Part model, mm, in its own coordinate system. Round coordinates to 2 decimals unless told otherwise and drop trailing zeros. Order: outer loops, then holes, each group sorted by start corner. A loop starts at its lowest first (then second) coordinate and runs counter-clockwise, first axis right, second up. Notation, with made-up numbers: (-31, 81.5) - (18, 81.5) arc R22 cw to (18, 109.5) - close; hole circle Ø5 at (79, 58). An arc over 180 degrees is marked (long way). Answer as a JSON object with one key per item and string values.
```python
from build123d import *

# Parameters (mm, degrees)
BOSS_EXTRUDE1_DEPTH = 4
SKETCH3_R           = 4
CUT_EXTRUDE1_DEPTH  = 105.985426706
FILLET1_R           = 5


with BuildPart() as part:
    # Sketch2 → Boss-Extrude1 (new body)
    with BuildSketch(Plane(origin=(0, 0, 0), x_dir=(1, 0, 0), z_dir=(0, 1, 0))):
        Polygon((70, -37.725994468), (70, -7.725994468), (0, 32.688524375), (0, -78.140513312), align=None)
    extrude(amount=BOSS_EXTRUDE1_DEPTH)

    # Sketch3 → Cut-Extrude1 (cut, through all)
    with BuildSketch(Plane(origin=(0, 4, 0), x_dir=(1, 0, 0), z_dir=(0, 1, 0))):
        with Locations(Location((55, -22.725994468, 0), (0, 0, 270))):
            Circle(SKETCH3_R)
    extrude(amount=-CUT_EXTRUDE1_DEPTH, mode=Mode.SUBTRACT)

    # Fillet1
    fillet1_edges = [part.edges().sort_by_distance(p)[0] for p in [
        (70, 2, 7.725994468),
        (70, 2, 37.725994468),
    ]]
    fillet(fillet1_edges, radius=FILLET1_R)


solid = part.part
```
Item 1: Cut at B-B (x = 55). Write the cut outline in (y, z).
Taken from the geometry:
{"outline": "(0, -0.93) - (4, -0.93) - (4, 18.73) - (0, 18.73) - close; (0, 26.73) - (4, 26.73) - (4, 46.39) - (0, 46.39) - close"}
Item 2: Cut at A-A (y = 2.7). Write the cut outline in (x, z).
Taken from the geometry:
{"outline": "(0, -32.69) - (67.5, 6.28) arc R5 ccw to (70, 10.61) - (70, 34.84) arc R5 ccw to (67.5, 39.17) - (0, 78.14) - close; hole circle Ø8 at (55, 22.73)"}
Item 3: Cut at C-C (z = -24.5). Write the cut outline in (x, y), plus the area to 3 significant figures.
Taken from the geometry:
{"outline": "(0, 0) - (14.18, 0) - (14.18, 4) - (0, 4) - close", "area": "56.7 mm2"}
Item 4: Probe L1, parallel to X at y = 0.2, z = 21.5; L2, parallel to Z at x = 51.5, y = 0.5; L3, parallel to Z at x = 23, y = 0.8. List the from-to ranges inside material, lowest first. Write a range as from..to.
Taken from the geometry:
{"L1": "0..51.19, 58.81..70", "L2": "-2.95..20.79, 24.66..48.41", "L3": "-19.41..64.86"}
Item 5: Cut at D-D (x = 25.5). Write the cut outline in (y, z).
Taken from the geometry:
{"outline": "(0, -17.97) - (4, -17.97) - (4, 63.42) - (0, 63.42) - close"}
Item 6: Drop flat-ended pins along their axis: P1, Ø7, axis at x = 55, z = 22.73, coming from the -Y side; P2, Ø1, axis at x = 44.5, y = 3, coming from the +Z side. Give the stop position or say it passes through.
Taken from the geometry:
{"P1": "through", "P2": "z = 52.74"}
Item 7: Two-plate mould, pull along Z, no slides. Class faces 1 (the cylindrical face through (51.095, 2.028, 21.859)), 2 (the cylindrical face through (69.348, 2.028, 8.145)), 3 (the flat face through (0, 2, 22)): pulls with the +Z half, pulls with the -Z half, needs draft (parallel to the pull), parting line crosses it, or undercut.
Taken from the geometry:
{"face 1": "undercut", "face 2": "pulls with the -Z half", "face 3": "needs draft"}
